Verification items for the finished model (mm, model axes). Round coordinates to 2 decimals unless told otherwise and drop trailing zeros. Write each loop counter-clockwise with the first axis right and the second up, starting at its lowest first coordinate (ties: lowest second). Pieces come first, ordered by that corner, then holes. Notation, with made-up numbers: M 4,12 L 58,12 A22 ccw 58,18 Z; hole C 33.25,68.5 d8. An arc over 180 degrees is marked long. One line per question, with ' | ' between items.
from build123d import *

# Parameters (mm, degrees)
SKETCH1_W           = 26
SKETCH1_H           = 18
BOSS_EXTRUDE1_DEPTH = 13
SKETCH2_R           = 1.35
CUT_EXTRUDE1_DEPTH  = 14
SKETCH3_W           = 26
SKETCH3_H           = 13.75
CUT_EXTRUDE3_DEPTH  = 14
SKETCH4_W           = 26
SKETCH4_H           = 10
CUT_EXTRUDE4_DEPTH  = 5.25


with BuildPart() as part:
    # Sketch1 → Boss-Extrude1 (new body)
    with BuildSketch(Plane(origin=(0, 0, 0), x_dir=(1, 0, 0), z_dir=(0, 1, 0))):
        with Locations((13, 9)):
            Rectangle(SKETCH1_W, SKETCH1_H)
    extrude(amount=BOSS_EXTRUDE1_DEPTH)

    # Sketch2 → Cut-Extrude1 (cut, through all)
    with BuildSketch(Plane(origin=(0, 13, 0), x_dir=(1, 0, 0), z_dir=(0, 1, 0))):
        with Locations((3, 15.25)):
            Circle(SKETCH2_R)
        with Locations((23, 15.25)):
            Circle(SKETCH2_R)
        with Locations((3, 2.75)):
            Circle(SKETCH2_R)
        with Locations((23, 2.75)):
            Circle(SKETCH2_R)
    extrude(amount=-CUT_EXTRUDE1_DEPTH, mode=Mode.SUBTRACT)

    # Sketch3 → Cut-Extrude3 (cut, through all)
    with BuildSketch(Plane(origin=(0, 13, 0), x_dir=(1, 0, 0), z_dir=(0, 1, 0))):
        with Locations((13, 11.125)):
            Rectangle(SKETCH3_W, SKETCH3_H)
    extrude(amount=-CUT_EXTRUDE3_DEPTH, mode=Mode.SUBTRACT)

    # Sketch4 → Cut-Extrude4 (cut, through all)
    with BuildSketch(Plane.XY):
        with Locations((13, 5)):
            Rectangle(SKETCH4_W, SKETCH4_H)
    extrude(amount=-CUT_EXTRUDE4_DEPTH, mode=Mode.SUBTRACT)


solid = part.part
1. Section check C-C, the plane y = 11.1. Record the cut outline in (x, z).
Results:
outline: M 0,-4.25 L 26,-4.25 L 26,0 L 0,0 Z; hole C 3,-2.75 d2.7; hole C 23,-2.75 d2.7
2. Mould release check, pull along X, two halves, no side actions. Record for faces 1 (the face through (26, 11, -2)), 2 (the face through (13, 10, -2)), 3 (the face through (3.62, 11.52, -1.55)): pulls with the +X half, pulls with the -X half, needs draft (parallel to the pull), parting line crosses it, or undercut.
Results:
face 1: pulls with the +X half | face 2: needs draft | face 3: undercut
3. Section check A-A, the plane z = -2.75. Record the cut outline in (x, y), then the cut area to 3 significant figures.
Results:
outline: M 0,10 L 1.65,10 L 1.65,13 L 0,13 Z; M 4.35,10 L 21.65,10 L 21.65,13 L 4.35,13 Z; M 24.35,10 L 26,10 L 26,13 L 24.35,13 Z | area: 61.8 mm2
4. Thickness scan on line 1 (X direction, y = 12.35, z = -2.75); line 2 (X direction, y = 10.9, z = -3.95); line 3 (Z direction, x = 23, y = 12.4). Record the ranges inside material, lowest first.
Results:
line 1: x = 0 to 1.65, 4.35 to 21.65, 24.35 to 26 | line 2: x = 0 to 2.38, 3.62 to 22.38, 23.62 to 26 | line 3: z = -4.25 to -4.1, -1.4 to 0
5. Section check B-B, the plane x = 23. Record the cut outline in (y, z), then the cut area to 3 significant figures.
Results:
outline: M 10,-4.25 L 13,-4.25 L 13,-4.1 L 10,-4.1 Z; M 10,-1.4 L 13,-1.4 L 13,0 L 10,0 Z | area: 4.65 mm2
